from build123d import *

# Parameters (mm, degrees)
PAD_DEPTH       = 4
PAD001_DEPTH    = 10
SKETCH002_R     = 5
PAD002_DEPTH    = 3
POCKET_DEPTH    = 3
SKETCH004_R     = 1.7
POCKET001_DEPTH = 4
POCKET002_DEPTH = 3
SKETCH006_R     = 1.7
POCKET003_DEPTH = 2
POCKET004_DEPTH = 3
SKETCH008_R     = 1.7
POCKET005_DEPTH = 2
POCKET006_DEPTH = 3
SKETCH010_R     = 1.7
POCKET007_DEPTH = 2
POCKET008_DEPTH = 3
SKETCH012_R     = 1.7
POCKET009_DEPTH = 2


with BuildPart() as part:
    # Sketch → Pad (new body)
    with BuildSketch(Plane.XY):
        with BuildLine():
            Line((0, 0), (42, 0))
            ThreePointArc((42, 0), (47.656854, 2.343146), (50, 8))
            Line((50, 62), (50, 8))
            ThreePointArc((50, 62), (47.656854, 67.656854), (42, 70))
            Line((42, 70), (0, 70))
            Line((0, 70), (0, 0))
        make_face()
    extrude(amount=PAD_DEPTH)

    # Sketch001 → Pad001 (new body)
    with BuildSketch(Plane.XY.offset(4)):
        with BuildLine():
            Line((0, 0), (42, 0))
            ThreePointArc((42, 0), (47.656854, 2.343146), (50, 8))
            Line((50, 62), (50, 8))
            ThreePointArc((50, 62), (47.656854, 67.656854), (42, 70))
            Line((42, 70), (0, 70))
            Line((0, 70), (0, 0))
        make_face()
        with BuildLine():
            ThreePointArc((48, 62), (46.242641, 66.242641), (42, 68))
            Line((42, 68), (24, 68))
            Line((24, 68), (24, 65))
            Line((24, 65), (16, 65))
            Line((16, 65), (16, 68))
            Line((16, 68), (2, 68))
            Line((2, 68), (2, 56.5))
            Line((2, 56.5), (5, 56.5))
            Line((5, 56.5), (5, 48.5))
            Line((5, 48.5), (2, 48.5))
            Line((2, 48.5), (2, 21.5))
            Line((2, 21.5), (5, 21.5))
            Line((5, 21.5), (5, 13.5))
            Line((5, 13.5), (2, 13.5))
            Line((2, 13.5), (2, 2))
            Line((2, 2), (16, 2))
            Line((16, 2), (16, 5))
            Line((16, 5), (24, 5))
            Line((24, 5), (24, 2))
            Line((24, 2), (42, 2))
            ThreePointArc((42, 2), (46.242641, 3.757359), (48, 8))
            Line((48, 31), (48, 8))
            Line((45, 31), (48, 31))
            Line((45, 39), (45, 31))
            Line((48, 39), (45, 39))
            Line((48, 62), (48, 39))
        make_face(mode=Mode.SUBTRACT)
    extrude(amount=PAD001_DEPTH)

    # Sketch002 → Pad002 (new body)
    with BuildSketch(Plane.XY.offset(4)):
        with Locations((28, 53)):
            Circle(SKETCH002_R)
        with Locations((42, 53)):
            Circle(SKETCH002_R)
        with Locations((28, 17)):
            Circle(SKETCH002_R)
        with Locations((42, 17)):
            Circle(SKETCH002_R)
    extrude(amount=PAD002_DEPTH)

    # Sketch003 → Pocket (cut)
    with BuildSketch(Plane.XY.offset(7)):
        Polygon((28, 50), (30.598076, 51.5), (30.598076, 54.5), (28, 56), (25.401924, 54.5), (25.401924, 51.5), align=None)
        Polygon((30.598076, 15.5), (30.598076, 18.5), (28, 20), (25.401924, 18.5), (25.401924, 15.5), (28, 14), align=None)
        Polygon((44.598076, 51.5), (44.598076, 54.5), (42, 56), (39.401924, 54.5), (39.401924, 51.5), (42, 50), align=None)
        Polygon((44.598076, 15.5), (44.598076, 18.5), (42, 20), (39.401924, 18.5), (39.401924, 15.5), (42, 14), align=None)
    extrude(amount=-POCKET_DEPTH, mode=Mode.SUBTRACT)

    # Sketch004 → Pocket001 (cut)
    with BuildSketch(Plane.XY.offset(4)):
        with Locations((28, 53)):
            Circle(SKETCH004_R)
        with Locations((42, 53)):
            Circle(SKETCH004_R)
        with Locations((28, 17)):
            Circle(SKETCH004_R)
        with Locations((42, 17)):
            Circle(SKETCH004_R)
    extrude(amount=-POCKET001_DEPTH, mode=Mode.SUBTRACT)

    # Sketch005 → Pocket002 (cut)
    with BuildSketch(Plane.YZ.offset(5)):
        Polygon((20.098076, 7.5), (20.098076, 10.5), (17.5, 12), (14.901924, 10.5), (14.901924, 7.5), (17.5, 6), align=None)
        Polygon((55.098076, 7.5), (55.098076, 10.5), (52.5, 12), (49.901924, 10.5), (49.901924, 7.5), (52.5, 6), align=None)
    extrude(amount=-POCKET002_DEPTH, mode=Mode.SUBTRACT)

    # Sketch006 → Pocket003 (cut)
    with BuildSketch(Plane.YZ.offset(2)):
        with Locations((17.5, 9)):
            Circle(SKETCH006_R)
        with Locations((52.5, 9)):
            Circle(SKETCH006_R)
    extrude(amount=-POCKET003_DEPTH, mode=Mode.SUBTRACT)

    # Sketch007 → Pocket004 (cut)
    with BuildSketch(Plane.XZ.offset(-65)):
        Polygon((22.598076, 7.5), (22.598076, 10.5), (20, 12), (17.401924, 10.5), (17.401924, 7.5), (20, 6), align=None)
    extrude(amount=-POCKET004_DEPTH, mode=Mode.SUBTRACT)

    # Sketch008 → Pocket005 (cut)
    with BuildSketch(Plane.XZ.offset(-68)):
        with Locations((20, 9)):
            Circle(SKETCH008_R)
    extrude(amount=-POCKET005_DEPTH, mode=Mode.SUBTRACT)

    # Sketch009 → Pocket006 (cut)
    with BuildSketch(Plane(origin=(45, 0, 0), x_dir=(0, -1, 0), z_dir=(-1, 0, 0))):
        Polygon((-37.598076, 7.5), (-35, 6), (-32.401924, 7.5), (-32.401924, 10.5), (-35, 12), (-37.598076, 10.5), align=None)
    extrude(amount=-POCKET006_DEPTH, mode=Mode.SUBTRACT)

    # Sketch010 → Pocket007 (cut)
    with BuildSketch(Plane(origin=(48, 0, 0), x_dir=(0, -1, 0), z_dir=(-1, 0, 0))):
        with Locations((-35, 9)):
            Circle(SKETCH010_R)
    extrude(amount=-POCKET007_DEPTH, mode=Mode.SUBTRACT)

    # Sketch011 → Pocket008 (cut)
    with BuildSketch(Plane(origin=(0, 5, 0), x_dir=(-1, 0, 0), z_dir=(0, 1, 0))):
        Polygon((-17.401924, 7.5), (-17.401924, 10.5), (-20, 12), (-22.598076, 10.5), (-22.598076, 7.5), (-20, 6), align=None)
    extrude(amount=-POCKET008_DEPTH, mode=Mode.SUBTRACT)

    # Sketch012 → Pocket009 (cut)
    with BuildSketch(Plane(origin=(0, 2, 0), x_dir=(-1, 0, 0), z_dir=(0, 1, 0))):
        with Locations((-20, 9)):
            Circle(SKETCH012_R)
    extrude(amount=-POCKET009_DEPTH, mode=Mode.SUBTRACT)


solid = part.part
Verification items for the finished model (mm, model axes). A direction names the side the tool comes from. Coordinates: 2 decimals unless noted, no trailing zeros. Order: outer loops, then holes, each group sorted by start corner. A loop starts at its lowest first (then second) coordinate and runs counter-clockwise, first axis right, second up. Notation, with made-up numbers: M 27.5,-14.5 L 51.5,-14.5 A12 cw 51.5,4.5 Z; hole C 51,19.5 d9. An arc over 180 degrees is marked long. One line per item, written item: value. Start each with the question number.
Item 1: Access from +Z, -Z, +X, -X, +Y, -Y to the whole of each face (thin tool, end or side, straight path). Record for faces 1 (the flat face through (3, 21.5, 9)), 2 (the flat face through (18.68, 66.48, 6.76)), 3 (the cylindrical face through (18.43, 1.01, 8.35)).
Item 2: Sectioned sample at D-D (x = 10.5). Enter the section's corners in (y, z), then the cut area to 3 significant figures.
Item 3: Mould release check, pull along X, two halves, no side actions. Record for faces 4 (the flat face through (9, 68, 9)), 5 (the flat face through (21, 70, 7)): released by +X, released by -X, zero draft, split by the parting line, or undercut.
Item 4: Gauge pin test, flat ends, axial feed: pin 1 (6 mm diameter, centred on x = 32.5, y = 16.5, fed in from +Z); pin 2 (1.6 mm diameter, centred on x = 41.5, y = 51.5, fed in from +Z). Record the tip position at first contact, or that the pin passes through.
Item 5: Scan lines: probe 1 along Y at (x, z) = (28, 1.95); probe 2 along X at (y, z) = (30.5, 12); probe 3 along Y at (x, z) = (27, 8). Record each from-to range of solid material in increasing order.
Item 6: Sectioned sample at B-B (y = 23.5). Enter the section's corners in (x, z).
Item 7: Sectioned sample at A-A (x = 41). Count the separate pieces of the cut face and the enclosed holes in it, then the cut area to 3 significant figures.
Conclusion:
1. face 1: +Z
1. face 2: none
1. face 3: +Y, -Y
2. outline: M 0,0 L 70,0 L 70,14 L 68,14 L 68,4 L 2,4 L 2,14 L 0,14 Z
2. area: 320 mm^2
3. face 4: undercut
3. face 5: zero draft
4. pin 1: stops at z = 7
4. pin 2: stops at z = 4
5. probe 1: y = 0 to 15.3, 18.7 to 51.3, 54.7 to 70
5. probe 2: x = 0 to 2, 48 to 50
5. probe 3: y = 0 to 2, 68 to 70
6. outline: M 0,0 L 50,0 L 50,14 L 48,14 L 48,4 L 2,4 L 2,14 L 0,14 Z
7. separate pieces: 3
7. enclosed holes: 0
7. area: 328 mm^2
